from build123d import *

# Parameters (mm, degrees)
SKETCH1_W           = 46.2
SKETCH1_H           = 12
BOSS_EXTRUDE1_DEPTH = 10
SKETCH2_W           = 4.6
SKETCH2_H           = 12
BOSS_EXTRUDE2_DEPTH = 7
SKETCH8_R           = 6
BOSS_EXTRUDE3_DEPTH = 4.6
LPATTERN1_COUNT     = 4
LPATTERN1_PITCH     = 9
SKETCH4_R           = 2.1
CUT_EXTRUDE1_DEPTH  = 39.9
SKETCH10_W          = 26
SKETCH10_H          = 12
BOSS_EXTRUDE4_DEPTH = 25
SKETCH11_W          = 19
SKETCH11_H          = 6
CUT_EXTRUDE2_DEPTH  = 25
FILLET1_R           = 3
FILLET2_R           = 0.5
SKETCH12_R          = 1.5
CUT_EXTRUDE3_DEPTH  = 10


with BuildPart() as part:
    # Sketch1 → Boss-Extrude1 (new body)
    with BuildSketch(Plane(origin=(0, 0, 0), x_dir=(1, 0, 0), z_dir=(0, 1, 0))):
        Rectangle(SKETCH1_W, SKETCH1_H)
    extrude(amount=BOSS_EXTRUDE1_DEPTH)

    # Sketch2 → Boss-Extrude2 (add)
    with BuildSketch(Plane.XZ):
        with Locations((13.5, 0)):
            Rectangle(SKETCH2_W, SKETCH2_H)
    boss_extrude2 = extrude(amount=BOSS_EXTRUDE2_DEPTH)

    # Sketch8 → Boss-Extrude3 (add)
    with BuildSketch(Plane(origin=(15.8, 0, 0), x_dir=(0, 0, -1), z_dir=(1, 0, 0))):
        with Locations((0, -7)):
            Circle(SKETCH8_R)
    boss_extrude3 = extrude(amount=-BOSS_EXTRUDE3_DEPTH)

    # LPattern1: Boss-Extrude2, Boss-Extrude3 ×4
    with Locations(*[(-i * LPATTERN1_PITCH, 0, 0) for i in range(1, LPATTERN1_COUNT)]):
        add(boss_extrude2)
        add(boss_extrude3)

    # Sketch4 → Cut-Extrude1 (cut, through all)
    with BuildSketch(Plane(origin=(15.8, 0, 0), x_dir=(0, 0, -1), z_dir=(1, 0, 0))):
        with Locations((0, -7)):
            Circle(SKETCH4_R)
    extrude(amount=-CUT_EXTRUDE1_DEPTH, mode=Mode.SUBTRACT)

    # Sketch10 → Boss-Extrude4 (add)
    with BuildSketch(Plane(origin=(0, 10, 0), x_dir=(1, 0, 0), z_dir=(0, 1, 0))):
        Rectangle(SKETCH10_W, SKETCH10_H)
    extrude(amount=BOSS_EXTRUDE4_DEPTH)

    # Sketch11 → Cut-Extrude2 (cut)
    with BuildSketch(Plane(origin=(0, 35, 0), x_dir=(1, 0, 0), z_dir=(0, 1, 0))):
        with Locations((0, 3)):
            Rectangle(SKETCH11_W, SKETCH11_H)
    extrude(amount=-CUT_EXTRUDE2_DEPTH, mode=Mode.SUBTRACT)

    # Fillet1
    fillet1_edges = [part.edges().sort_by_distance(p)[0] for p in [
        (-13, 10, 0),
        (13, 10, 0),
        (23.1, 10, 0),
        (-23.1, 10, 0),
    ]]
    fillet(fillet1_edges, radius=FILLET1_R)

    # Fillet2
    fillet2_edges = [part.edges().sort_by_distance(p)[0] for p in [
        (-13, 35, 0),
        (0, 35, 6),
        (13, 35, 0),
        (11.25, 35, -6),
        (-11.25, 35, -6),
        (-9.5, 35, -3),
        (0, 35, 0),
        (9.5, 35, -3),
    ]]
    fillet(fillet2_edges, radius=FILLET2_R)

    # Sketch12 → Cut-Extrude3 (cut, symmetric)
    with BuildSketch(Plane.XY):
        with Locations((0, 17.5)):
            Circle(SKETCH12_R)
        with Locations((0, 27.5)):
            Circle(SKETCH12_R)
    extrude(amount=CUT_EXTRUDE3_DEPTH, both=True, mode=Mode.SUBTRACT)


solid = part.part
The listing builds one solid part. Answer for the finished solid, in the listing's coordinates (mm). A direction names the side the tool comes from. Round coordinates to 2 decimals unless told otherwise and drop trailing zeros. Loops run counter-clockwise (first coordinate to the right, second up) from the corner with the lowest first, then second, coordinate; pieces in that order, holes last. Notation, with made-up numbers: M -33.75,10 L -10.75,10 A29 cw -10.75,34 Z; hole C 12.25,-21 d7. An arc over 180 degrees is marked long. Return JSON: item names as keys, results as strings.
Q1. Find section C-C, the plane z = 3. State how many separate pieces and enclosed holes the cut face has, plus the area to 3 significant figures.
Results list:
{"separate pieces": "1", "enclosed holes": "2", "area": "1,320 mm2"}
Q2. Find section A-A, the plane y = 27.5. Determine the outline of the cut face in (x, z), plus the area to 3 significant figures.
Results list:
{"outline": "M -13,-6 L -9.5,-6 L -9.5,0 L -1.5,0 L -1.5,6 L -13,6 Z; M 1.5,0 L 9.5,0 L 9.5,-6 L 13,-6 L 13,6 L 1.5,6 Z", "area": "180 mm2"}
Q3. Which of the six approach directions +Z, -Z, +X, -X, +Y, -Y give full straight-line access (tool end or side, diameter ignored) to faces 5 (the face through (2.2, -5, -1.2)), 6 (the face through (18, 10, 0)), 7 (the face through (9.5, 22, -3)), 8 (the face through (-20, 0, 0))?
Results list:
{"face 5": "+Z, -Z, -Y", "face 6": "+Z, -Z, +X, +Y", "face 7": "-Z, +Y", "face 8": "+Z, -Z, -X, -Y"}
Q4. Each of these flat-tipped pins is pushed along its axis until it touches: pin 1 Ø2 at (x, z) = (18, -1.5) entering from -Y; pin 2 Ø6.5 at (x, z) = (3.5, -4) entering from +Y; pin 3 Ø5.5 at (x, y) = (0.5, 22) entering from -Z. Where does it stop, or does it pass through?
Results list:
{"pin 1": "stops at y = 0", "pin 2": "stops at y = 10", "pin 3": "stops at z = 0"}
Q5. Find section B-B, the plane x = -3.5. Determine the outline of the cut face in (y, z).
Results list:
{"outline": "M -7,-6 L 10,-6 L 10,0 L 34.5,0 A0.5 ccw 35,0.5 L 35,5.5 A0.5 ccw 34.5,6 L -7,6 A6 ccw Z; hole C -7,0 d4.2"}
Q6. Find section D-D, the plane x = -15. Determine the outline of the cut face in (y, z), plus the area to 3 significant figures.
Results list:
{"outline": "M -7,-6 L 10.17,-6 L 10.17,6 L -7,6 A6 ccw Z; hole C -7,0 d4.2", "area": "249 mm2"}
Q7. Find the intervals of material crossed by line 1 along Y through (x, z) = (0, 4.1); line 2 along X through (y, z) = (26, -4.75); line 3 along Y through (x, z) = (-14.7, 0), in increasing order. Write a range as from..to.
Results list:
{"line 1": "y = 0..16, 19..26, 29..35", "line 2": "x = -13..-9.5, 9.5..13", "line 3": "y = -13..-9.1, -4.9..10.3"}
Q8. The mould has two halves that part along X. Classify faces 1 (the face through (13.86, 10.9, -0.08)), 2 (the face through (0, 10, -3)), 3 (the face through (-4.468, -4.918, 0.273)), 4 (the face through (-13.9, 10.86, -0.08)): released by +X, released by -X, zero draft, split by the parting line, or undercut.
Results list:
{"face 1": "released by +X", "face 2": "undercut", "face 3": "zero draft", "face 4": "released by -X"}
